CAD build for the part. Positions are in the model's coordinates, mm. A direction names the side the tool comes from. Round coordinates to 2 decimals unless told otherwise and drop trailing zeros. Loops run counter-clockwise (first coordinate to the right, second up) from the corner with the lowest first, then second, coordinate; pieces in that order, holes last. Notation, with made-up numbers: (49, 88) -> (64, 88) arc R28 ccw to (64, 112) -> close; hole circle Ø5 at (77, 71.25). An arc over 180 degrees is marked (long way). Answer as CSV lines item,"result".
Autodesk Inventor part; units mm, degrees
ref_plane "YZ Plane" through (0, 0, 0) normal (1, 0, 0) x (0, 1, 0)
ref_plane "XZ Plane" through (0, 0, 0) normal (0, 1, 0) x (-1, 0, 0)
ref_plane "XY Plane" through (0, 0, 0) normal (0, 0, 1) x (1, 0, 0)
sketch "Sketch1" plane through (0, 0, 0) normal (0, 0, 1) x (1, 0, 0)
  circle A0 centre (-0.6115, -1.5992) radius 3.175
  line L0 (-6.0374, -1.5992) -> (-3.3244, 3.0998)
  line L1 (-3.3244, 3.0998) -> (2.1015, 3.0998)
  line L2 (2.1015, 3.0998) -> (4.8145, -1.5992)
  line L3 (4.8145, -1.5992) -> (2.1015, -6.2982)
  line L4 (2.1015, -6.2982) -> (-3.3244, -6.2982)
  line L5 (-3.3244, -6.2982) -> (-6.0374, -1.5992)
  dimension "d10" = 9.398
extrude "Extrusion1" add sketch "Sketch1" against normal blind 63.5 contours A0
extrude "Extrusion2" add sketch "Sketch1" along normal blind 4.699 contours A0 | L0 L1 L2 L3 L4 L5
thread "Thread1"
properties part number "HW-00063"
Q1. Tool access for faces 1 (the cylindrical face through (-3.13, -3.53, -31.31)), 2 (the flat face through (-1, -2, 4.699)): list every direction of +Z, -Z, +X, -X, +Y, -Y with a clear straight run to the whole face (end or side of a thin tool).
Results:
face 1,"-Z"
face 2,"+Z, +X, -X, +Y, -Y"
Q2. Probe L1, parallel to Z at x = 1.25, y = 2.75; L2, parallel to X at y = -2.25, z = -17.5; L3, parallel to Y at x = -0.5, z = -10.5. List the from-to ranges inside material, lowest first. Write a range as [from, to].
Results:
L1,"[0, 4.7]"
L2,"[-3.72, 2.5]"
L3,"[-4.77, 1.57]"
Q3. Drop flat-ended pins along their axis: pin 1 Ø1.5 at (y, z) = (-2.5, -16.5) entering from +X; pin 2 Ø1 at (y, z) = (-3, -29) entering from +X; pin 3 Ø3 at (y, z) = (1.5, -48) entering from -X. Give the stop position or say it passes through.
Results:
pin 1,"x = 2.56"
pin 2,"x = 2.43"
pin 3,"x = -3.35"
Q4. Slice it at A-A, the plane y = 0.75. Give the cut face in (x, z), and give its area (4 significant figures).
Results:
outline,"(-4.68, 0) -> (-2.75, 0) -> (-2.75, -63.5) -> (1.52, -63.5) -> (1.52, 0) -> (3.46, 0) -> (3.46, 4.7) -> (-4.68, 4.7) -> close"
area,"309.5 mm2"
Q5. Slice it at D-D, the plane x = 3.75. Give the cut face in (y, z).
Results:
outline,"(-3.44, 0) -> (0.24, 0) -> (0.24, 4.7) -> (-3.44, 4.7) -> close"
Q6. Slice it at B-B, the plane x = -2.75. Give the cut face in (y, z).
Results:
outline,"(-6.3, 0) -> (-3.95, 0) -> (-3.95, -63.5) -> (0.75, -63.5) -> (0.75, 0) -> (3.1, 0) -> (3.1, 4.7) -> (-6.3, 4.7) -> close"
